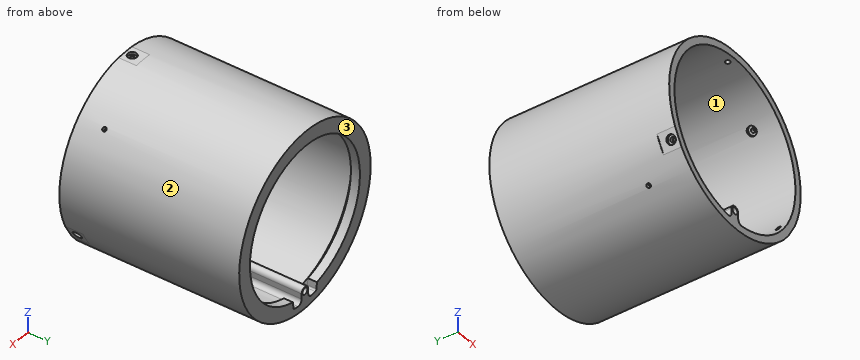
```python
from build123d import *

# Parameters (mm, degrees)
SCHIZZO1_R                                           = 100
ESTRUSIONE_ESTRUSIONE1_DEPTH                         = 200
RACCORDO1_R                                          = 5
ESTRUSIONE_ESTRUSIONE2_START                         = -10
ESTRUSIONE_ESTRUSIONE2_DEPTH                         = 10
SMUSSO1_START                                        = 184.4999999
SMUSSO1_DEPTH                                        = 5.5000001
SMUSSO1_2_ANGLE                                      = 338.362808
RACCORDO2_R                                          = 2.113506
SCHIZZO6_R                                           = 3.75
TAGLIO_ESTRUSIONE1_DEPTH                             = 200
TAGLIO_ESTRUSIONE2_DEPTH                             = 20
FORO_LAMATO_PER_BULLONE_M5_A_TESTA_ESAGO_D           = 5.4
FORO_LAMATO_PER_BULLONE_M5_A_TESTA_ESAGO_DEPTH       = 30
FORO_LAMATO_PER_BULLONE_M5_A_TESTA_ESAGO_CBORE_D     = 10
FORO_LAMATO_PER_BULLONE_M5_A_TESTA_ESAGO_CBORE_DEPTH = 3
FORO_LAMATO_PER_BULLONE_M5_A_TESTA_ESAGO_TIP         = 1.622323671
FORO_LAMATO_PER_BULLONE_M5_A_TESTA_E_2_D             = 5.4
FORO_LAMATO_PER_BULLONE_M5_A_TESTA_E_2_DEPTH         = 30
FORO_LAMATO_PER_BULLONE_M5_A_TESTA_E_2_CBORE_D       = 10
FORO_LAMATO_PER_BULLONE_M5_A_TESTA_E_2_CBORE_DEPTH   = 3
FORO_LAMATO_PER_BULLONE_M5_A_TESTA_E_2_TIP           = 1.622323671
FORO_LAMATO_PER_BULLONE_M5_A_TESTA_E_3_D             = 5.4
FORO_LAMATO_PER_BULLONE_M5_A_TESTA_E_3_DEPTH         = 30
FORO_LAMATO_PER_BULLONE_M5_A_TESTA_E_3_CBORE_D       = 10
FORO_LAMATO_PER_BULLONE_M5_A_TESTA_E_3_CBORE_DEPTH   = 3
FORO_LAMATO_PER_BULLONE_M5_A_TESTA_E_3_TIP           = 1.622323671
FORO_LAMATO_PER_VITE_M4_A_TESTA_ESAGONAL_D           = 4.5
FORO_LAMATO_PER_VITE_M4_A_TESTA_ESAGONAL_DEPTH       = 30
FORO_LAMATO_PER_VITE_M4_A_TESTA_ESAGONAL_CBORE_D     = 10
FORO_LAMATO_PER_VITE_M4_A_TESTA_ESAGONAL_CBORE_DEPTH = 3
FORO_LAMATO_PER_VITE_M4_A_TESTA_ESAGONAL_TIP         = 1.351936393
FORO_LAMATO_PER_VITE_M4_A_TESTA_ESAG_2_D             = 4.5
FORO_LAMATO_PER_VITE_M4_A_TESTA_ESAG_2_DEPTH         = 30
FORO_LAMATO_PER_VITE_M4_A_TESTA_ESAG_2_CBORE_D       = 10
FORO_LAMATO_PER_VITE_M4_A_TESTA_ESAG_2_CBORE_DEPTH   = 3
FORO_LAMATO_PER_VITE_M4_A_TESTA_ESAG_2_TIP           = 1.351936393


with BuildPart() as part:
    # Schizzo1 → Estrusione-Estrusione1 (new body)
    with BuildSketch(Plane(origin=(0, 0, 0), x_dir=(1, 0, 0), z_dir=(0, 1, 0))):
        with Locations(Location((0, 0, 0), (0, 0, 270))):
            Circle(SCHIZZO1_R)
        with BuildLine():
            Line((-5, 80.409122957), (-5, 91.864029957))
            ThreePointArc((-5, 91.864029957), (0, -92), (5, 91.864029957))
            Line((5, 91.864029957), (5, 80.409122957))
            ThreePointArc((5, 80.409122957), (0, 75.409122957), (-5, 80.409122957))
        make_face(mode=Mode.SUBTRACT)
    extrude(amount=ESTRUSIONE_ESTRUSIONE1_DEPTH)

    # Raccordo1
    raccordo1_edges = [part.edges().sort_by_distance(p)[0] for p in [
        (-5, 100, -91.864029957),
        (5, 100, -91.864029957),
    ]]
    fillet(raccordo1_edges, radius=RACCORDO1_R)

    # Schizzo2 → Estrusione-Estrusione2 (add)
    with BuildSketch(Plane(origin=(0, 200, 0), x_dir=(1, 0, 0), z_dir=(0, 1, 0)).offset(ESTRUSIONE_ESTRUSIONE2_START)):
        with BuildLine():
            ThreePointArc((18.3, 81.674965565), (0, -83.7), (-18.3, 81.674965565))
            Line((-18.3, 81.674965565), (-17.268411156, 90.364827096))
            ThreePointArc((-17.268411156, 90.364827096), (-58.631502512, -70.89673415), (92, 0))
            ThreePointArc((92, 0), (70.89673415, 58.631502512), (17.268411156, 90.364827096))
            Line((17.268411156, 90.364827096), (18.3, 81.674965565))
        make_face()
    extrude(amount=ESTRUSIONE_ESTRUSIONE2_DEPTH)

    # Smusso1: read off the stored shape, not the designer's step
    # Smusso1 outline → Smusso1 (add)
    with BuildSketch(Plane(origin=(0, 0, 0), x_dir=(1, 0, 0), z_dir=(0, 1, 0)).offset(SMUSSO1_START)):
        with BuildLine():
            Line((17.268411156, 90.364827097), (18.3, 81.674965565))
            ThreePointArc((18.3, 81.674965565), (0, -83.7), (-18.3, 81.674965565))
            Line((-18.3, 81.674965565), (-17.268411156, 90.364827097))
            ThreePointArc((-17.268411156, 90.364827097), (0, -92), (17.268411156, 90.364827097))
        make_face()
    extrude(amount=SMUSSO1_DEPTH)

    # Smusso1 2 outline → Smusso1 2 (revolve, cut)
    with BuildSketch(Plane(origin=(0, 0, 0), x_dir=(-0.18770012126264535, 0, -0.9822263814813712), z_dir=(0.9822263814813712, 0, -0.18770012126264535))):
        Polygon((92, 184.5), (83.7, 189.98740256), (83.7, 184.4999999), align=None)
    revolve(axis=Axis((0, 0, 0), (0, 1, 0)), revolution_arc=SMUSSO1_2_ANGLE, mode=Mode.SUBTRACT)

    # Raccordo2
    raccordo2_edges = [part.edges().sort_by_distance(p)[0] for p in [
        (17.268411156, 195, -90.364827096),
        (-17.268411156, 195, -90.364827096),
    ]]
    fillet(raccordo2_edges, radius=RACCORDO2_R)

    # Schizzo6 → Taglio-Estrusione1 (cut)
    with BuildSketch(Plane.XZ):
        with Locations(Location((0, -80.409122957, 0), (0, 0, 270))):
            Circle(SCHIZZO6_R)
    extrude(amount=-TAGLIO_ESTRUSIONE1_DEPTH, mode=Mode.SUBTRACT)

    # Schizzo7 → Taglio-Estrusione2 (cut)
    with BuildSketch(Plane.XZ):
        with BuildLine():
            ThreePointArc((10, 99.498743711), (0, 100), (-10, 99.498743711))
            Line((-10, 99.498743711), (10, 99.498743711))
        make_face()
        with BuildLine():
            ThreePointArc((81.168439698, -58.409625893), (86.602540378, -50), (91.168439698, -41.089117817))
            Line((91.168439698, -41.089117817), (81.168439698, -58.409625893))
        make_face()
        with BuildLine():
            Line((-81.168439698, -58.409625893), (-91.168439698, -41.089117817))
            ThreePointArc((-91.168439698, -41.089117817), (-86.602540378, -50), (-81.168439698, -58.409625893))
        make_face()
    extrude(amount=-TAGLIO_ESTRUSIONE2_DEPTH, mode=Mode.SUBTRACT)

    # Foro lamato per Bullone M5 a testa esago
    with Locations(Plane(origin=(86.168439698, 0, -49.749371855), x_dir=(-0.4999999999999976, 0, -0.86602540378444), z_dir=(0.8660254037844402, 0, -0.4999999999999977))):
        with Locations((0, 10)):
            CounterBoreHole(FORO_LAMATO_PER_BULLONE_M5_A_TESTA_ESAGO_D / 2, FORO_LAMATO_PER_BULLONE_M5_A_TESTA_ESAGO_CBORE_D / 2, FORO_LAMATO_PER_BULLONE_M5_A_TESTA_ESAGO_CBORE_DEPTH, depth=FORO_LAMATO_PER_BULLONE_M5_A_TESTA_ESAGO_DEPTH)
            with Locations((0, 0, -(FORO_LAMATO_PER_BULLONE_M5_A_TESTA_ESAGO_DEPTH + FORO_LAMATO_PER_BULLONE_M5_A_TESTA_ESAGO_TIP / 2))):  # 118° drill point
                Cone(0, FORO_LAMATO_PER_BULLONE_M5_A_TESTA_ESAGO_D / 2, FORO_LAMATO_PER_BULLONE_M5_A_TESTA_ESAGO_TIP, mode=Mode.SUBTRACT)

    # Foro lamato per Bullone M5 a testa e 2
    with Locations(Plane(origin=(-86.168439698, 0, -49.749371855), x_dir=(-0.5000000000000044, 0, 0.8660254037844362), z_dir=(-0.8660254037844362, 0, -0.5000000000000044))):
        with Locations((0, 8)):
            CounterBoreHole(FORO_LAMATO_PER_BULLONE_M5_A_TESTA_E_2_D / 2, FORO_LAMATO_PER_BULLONE_M5_A_TESTA_E_2_CBORE_D / 2, FORO_LAMATO_PER_BULLONE_M5_A_TESTA_E_2_CBORE_DEPTH, depth=FORO_LAMATO_PER_BULLONE_M5_A_TESTA_E_2_DEPTH)
            with Locations((0, 0, -(FORO_LAMATO_PER_BULLONE_M5_A_TESTA_E_2_DEPTH + FORO_LAMATO_PER_BULLONE_M5_A_TESTA_E_2_TIP / 2))):  # 118° drill point
                Cone(0, FORO_LAMATO_PER_BULLONE_M5_A_TESTA_E_2_D / 2, FORO_LAMATO_PER_BULLONE_M5_A_TESTA_E_2_TIP, mode=Mode.SUBTRACT)

    # Foro lamato per Bullone M5 a testa e 3
    with Locations(Plane.XY.offset(99.498743711)):
        with Locations((0, 8)):
            CounterBoreHole(FORO_LAMATO_PER_BULLONE_M5_A_TESTA_E_3_D / 2, FORO_LAMATO_PER_BULLONE_M5_A_TESTA_E_3_CBORE_D / 2, FORO_LAMATO_PER_BULLONE_M5_A_TESTA_E_3_CBORE_DEPTH, depth=FORO_LAMATO_PER_BULLONE_M5_A_TESTA_E_3_DEPTH)
            with Locations((0, 0, -(FORO_LAMATO_PER_BULLONE_M5_A_TESTA_E_3_DEPTH + FORO_LAMATO_PER_BULLONE_M5_A_TESTA_E_3_TIP / 2))):  # 118° drill point
                Cone(0, FORO_LAMATO_PER_BULLONE_M5_A_TESTA_E_3_D / 2, FORO_LAMATO_PER_BULLONE_M5_A_TESTA_E_3_TIP, mode=Mode.SUBTRACT)

    # Foro lamato per Vite M4 a testa esagonale-1
    with Locations(Plane(origin=(65.801169357, 29.385293, 64.297792429), x_dir=(0.698889048141, 0, -0.715230101707), z_dir=(-0.715230101707, 0, -0.698889048141))):
        with Locations((0, 0)):
            CounterBoreHole(FORO_LAMATO_PER_VITE_M4_A_TESTA_ESAGONAL_D / 2, FORO_LAMATO_PER_VITE_M4_A_TESTA_ESAGONAL_CBORE_D / 2, FORO_LAMATO_PER_VITE_M4_A_TESTA_ESAGONAL_CBORE_DEPTH, depth=FORO_LAMATO_PER_VITE_M4_A_TESTA_ESAGONAL_DEPTH)
            with Locations((0, 0, -(FORO_LAMATO_PER_VITE_M4_A_TESTA_ESAGONAL_DEPTH + FORO_LAMATO_PER_VITE_M4_A_TESTA_ESAGONAL_TIP / 2))):  # 118° drill point
                Cone(0, FORO_LAMATO_PER_VITE_M4_A_TESTA_ESAGONAL_D / 2, FORO_LAMATO_PER_VITE_M4_A_TESTA_ESAGONAL_TIP, mode=Mode.SUBTRACT)

    # Foro lamato per Vite M4 a testa esag 2
    with Locations(Plane(origin=(-62.673817972, 46.161135949, -67.349777585), x_dir=(0.732062968471, 0, -0.68123697066), z_dir=(0.68123697066, 0, 0.732062968471))):
        with Locations((0, 0)):
            CounterBoreHole(FORO_LAMATO_PER_VITE_M4_A_TESTA_ESAG_2_D / 2, FORO_LAMATO_PER_VITE_M4_A_TESTA_ESAG_2_CBORE_D / 2, FORO_LAMATO_PER_VITE_M4_A_TESTA_ESAG_2_CBORE_DEPTH, depth=FORO_LAMATO_PER_VITE_M4_A_TESTA_ESAG_2_DEPTH)
            with Locations((0, 0, -(FORO_LAMATO_PER_VITE_M4_A_TESTA_ESAG_2_DEPTH + FORO_LAMATO_PER_VITE_M4_A_TESTA_ESAG_2_TIP / 2))):  # 118° drill point
                Cone(0, FORO_LAMATO_PER_VITE_M4_A_TESTA_ESAG_2_D / 2, FORO_LAMATO_PER_VITE_M4_A_TESTA_ESAG_2_TIP, mode=Mode.SUBTRACT)


solid = part.part
```
Model file for the job. Use its own axes, mm. Face numbers are marked on the shaded views. Give positions to 0.01 mm unless a question says otherwise; leave off trailing zeros. Loops run counter-clockwise (first coordinate to the right, second up) from the corner with the lowest first, then second, coordinate; pieces in that order, holes last. Notation, with made-up numbers: (52, 26) - (61, 26) arc R5 cw to (61, 33) - close; hole circle Ø6 at (38.25, -4.5). An arc over 180 degrees is marked (long way). One line per item, written item: value. Start each with the question number.
1. Slice it at A-A (z = 0). List the corners of the cut face in (x, y), plus the area to 3 significant figures.
2. Probe L1, parallel to X at y = 125, z = 0; L2, parallel to Y at x = 0, z = 97; L3, parallel to Z at x = 2, y = 43. List the from-to ranges inside material, lowest first. Write a range as from..to.
3. Slice it at B-B (y = 165). List the corners of the cut face in (x, z), plus the area to 3 significant figures.
4. Pull direction X, two halves, no side cores. Call the marked faces 1, 2 and 3: pulls with the +X half, pulls with the -X half, needs draft (parallel to the pull), parting line crosses it, or undercut.
5. Pin check, flat tips, straight feed: pin 1 (6.5 mm diameter, centred on y = 52.5, z = -84.5, fed in from +X); pin 2 (5 mm diameter, centred on y = 78.5, z = -24, fed in from -X); pin 3 (5 mm diameter, centred on y = 155, z = -42.5, fed in from -X). Stop position of each tip, or through.
Solution:
1. outline: (-100, 0) - (-92, 0) - (-92, 184.5) - (-83.7, 189.99) - (-83.7, 200) - (-100, 200) - close; (83.7, 189.99) - (92, 184.5) - (92, 0) - (100, 0) - (100, 200) - (83.7, 200) - close
1. area: 3,410 mm^2
2. L1: x = -100..-92, 92..100
2. L2: y = 0..3, 13..200
2. L3: z = -99.98..-83.58, -77.24..-75.83, 91.98..99.98
3. outline: circle Ø200 at (0, 0); hole (-10.57, -91.39) arc R5 ccw to (-5, -86.42) - (-5, -80.41) arc R5 cw to (5, -80.41) - (5, -86.42) arc R5 ccw to (10.57, -91.39) arc R92 ccw (long way) to start; hole circle Ø7.5 at (0, -80.41)
3. area: 4,950 mm^2
4. face 1: undercut
4. face 2: parting line crosses it
4. face 3: needs draft
5. pin 1: stops at x = 58.3
5. pin 2: stops at x = -97.66
5. pin 3: stops at x = -91.65
